Read the model definition and answer for the solid it produces. Units are mm, in the model's axes. Give positions to 0.01 mm unless a question says otherwise; leave off trailing zeros. Loops run counter-clockwise (first coordinate to the right, second up) from the corner with the lowest first, then second, coordinate; pieces in that order, holes last. Notation, with made-up numbers: M 78,9 L 87,9 A20 cw 87,32 Z; hole C 8,78 d1. An arc over 180 degrees is marked long. Return JSON: item names as keys, results as strings. Group by question number.
```python
from build123d import *

# Parameters (mm, degrees)
F1_DEPTH = 25.4
F2_SIZE  = 0.635


with BuildPart() as f1:
    # F0 (on Right) → F1 (new body, symmetric)
    with BuildSketch(Plane.YZ):
        Polygon((-0.4185124813, 3.1472960304), (-1.9360904558, 2.5163820749), (-2.9348945562, 1.2112055746), (-3.1472960304, -0.4185124813), (-2.5163820749, -1.9360904558), (-1.2112055746, -2.9348945562), (0.4185124813, -3.1472960304), (1.9360904558, -2.5163820749), (2.9348945562, -1.2112055746), (3.1472960304, 0.4185124813), (2.5163820749, 1.9360904558), (1.2112055746, 2.9348945562), align=None)
    extrude(amount=F1_DEPTH, both=True)

    # F2
    f2_edges = [f1.edges().sort_by_distance(p)[0] for p in [
        (25.4, 1.177301, -2.831839),
        (25.4, 2.435493, -1.863794),
        (25.4, 3.041095, -0.396347),
        (25.4, 2.831839, 1.177301),
        (25.4, 1.863794, 2.435493),
        (25.4, 0.396347, 3.041095),
        (25.4, -1.177301, 2.831839),
        (25.4, -2.435493, 1.863794),
        (25.4, -3.041095, 0.396347),
        (25.4, -2.831839, -1.177301),
        (25.4, -1.863794, -2.435493),
        (25.4, -0.396347, -3.041095),
        (-25.4, 1.177301, -2.831839),
        (-25.4, 2.435493, -1.863794),
        (-25.4, 3.041095, -0.396347),
        (-25.4, 2.831839, 1.177301),
        (-25.4, 1.863794, 2.435493),
        (-25.4, 0.396347, 3.041095),
        (-25.4, -1.177301, 2.831839),
        (-25.4, -2.435493, 1.863794),
        (-25.4, -3.041095, 0.396347),
        (-25.4, -2.831839, -1.177301),
        (-25.4, -1.863794, -2.435493),
        (-25.4, -0.396347, -3.041095),
    ]]
    chamfer(f2_edges, length=F2_SIZE)


solid = f1.part
```
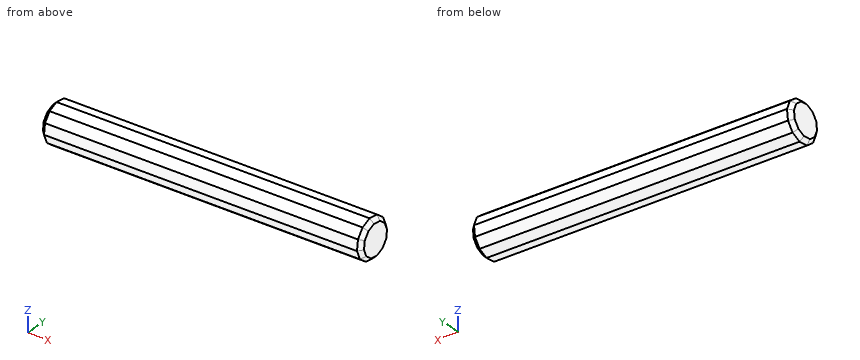
1. A flat-ended cylindrical pin translates along its axis: P1, Ø1.5, axis at x = 19, z = 2, coming from the -Y side. Find the tip coordinate at first contact, or state that the pin passes through.
2. Straight lines are drawn through the part: line 1 along Z through (x, y) = (-3, -0.25); line 2 along Z through (x, y) = (-7, -2); line 3 along X through (y, z) = (2, 2.25). For each, find the intervals that lie inside material, in ascending order.
3. Find section A-A (x = -10). Write down the section's boundary in (y, z).
Result:
{
 "1": {"P1": "stops at y = -2.91"},
 "2": {"line 1": "z = -3.06 to 3.13", "line 2": "z = -2.33 to 2.43", "line 3": "x = -24.83 to 24.83"},
 "3": {"outline": "M -3.15,-0.42 L -2.52,-1.94 L -1.21,-2.93 L 0.42,-3.15 L 1.94,-2.52 L 2.93,-1.21 L 3.15,0.42 L 2.52,1.94 L 1.21,2.93 L -0.42,3.15 L -1.94,2.52 L -2.93,1.21 Z"}
}
